Autodesk Fusion 360 part; units mm, degrees
sketch "Sketch1" plane through (0, 0, 0) normal (0, 0, 1) x (1, 0, 0)
  line L0 (-35, 30) -> (60, 30)
  line L1 (60, 30) -> (60, -52)
  line L2 (60, -52) -> (-35, -52)
  line L3 (-35, -52) -> (-35, 30)
  line L4 (-38, 33) -> (63, 33)
  line L5 (63, 33) -> (63, -55)
  line L6 (63, -55) -> (-38, -55)
  line L7 (-38, -55) -> (-38, 33)
  dimension "d1" = 82
  dimension "d2" = 95
  dimension "d3" = 3
  dimension "d4" = 3
  dimension "d5" = 3
  dimension "d6" = 3
extrude "Extrude1" add sketch "Sketch1" along normal blind 40
extrude "Extrude2" add sketch "Sketch1" along normal blind 4 contours L0 L1 L2 L3
sketch "Sketch2" plane through (63, 0, 0) normal (1, 0, 0) x (0, 1, 0)
  line L0 (-55, 0) -> (33, 0)
  line L1 (33, 0) -> (33, 40)
  line L2 (33, 40) -> (-55, 40)
  line L3 (-55, 40) -> (-55, 0)
  line L4 (-22, 29) -> (-40, 29)
  line L5 (-40, 29) -> (-40, 11)
  line L6 (-40, 11) -> (-22, 11)
  line L7 (-22, 11) -> (-22, 29)
  line L8 (-22, 29) -> (-40, 11) construction
  line L9 (-40, 29) -> (-22, 11) construction
  point P0 (-31, 20)
  dimension "d11" = 18
  dimension "d12" = 18
  dimension "d13" = 15
  dimension "d14" = 11
extrude "Extrude3" cut sketch "Sketch2" against normal blind 3 contours L4 L5 L6 L7
fillet "Fillet1" radius 2 1 edges at (63, -55, 20)
fillet "Fillet2" radius 2 1 edges at (63, 33, 20)
fillet "Fillet3" radius 2 1 edges at (-38, 33, 20)
fillet "Fillet4" radius 2 1 edges at (-38, -55, 20)
fillet "Fillet5" radius 2 1 edges at (-35, 30, 22)
fillet "Fillet6" radius 2 1 edges at (-35, -52, 22)
fillet "Fillet7" radius 2 1 edges at (60, -52, 22)
fillet "Fillet8" radius 2 1 edges at (60, 30, 22)
Geometry check sheet. Reference: the model listing, model coordinates, mm. A direction names the side the tool comes from. Coordinates: 2 decimals unless noted, no trailing zeros. Loops run counter-clockwise (first coordinate to the right, second up) from the corner with the lowest first, then second, coordinate; pieces in that order, holes last. Notation, with made-up numbers: (-31.75, -16.5) - (-2.75, -16.5) arc R37 cw to (-2.75, 22.5) - close; hole circle Ø9 at (-22, -38). An arc over 180 degrees is marked (long way). One line per item, written item: value. Start each with the question number.
(1) Tool access check on faces 1 (the flat face through (12, -10, 4)), 2 (the flat face through (62, -40, 20)), 3 (the flat face through (13, -55, 20)). Record the directions out of +Z, -Z, +X, -X, +Y, -Y that give a thin tool (end or side, any length) a straight path to the whole face; none if there is none.
(2) Cross-section at B-B on y = -36. Enter the section's corners in (x, z).
(3) Material ranges on line 1 (Y direction, x = -9, z = 20); line 2 (X direction, y = 4, z = 8); line 3 (Z direction, x = -33, y = -43.5), recorded low to high. Write a range as [from, to].
(4) Cross-section at C-C on x = -22. Enter the section's corners in (y, z).
(5) Depth check by flat-ended pin: P1, Ø10, axis at x = 44, y = -27.5, coming from the +Z side; P2, Ø0.9, axis at x = 62, z = 16, coming from the -Y side. Enter the tip coordinate at first touch or a pass-through.
(6) Mould release check, pull along X, two halves, no side actions. Record for faces 4 (the flat face through (62, -22, 20)), 5 (the flat face through (13, -52, 22)), 6 (the flat face through (-38, -12, 20)), 7 (the flat face through (63, -10, 20)): released by +X, released by -X, zero draft, split by the parting line, or undercut.
(7) Cross-section at D-D on y = 12.5. Enter the section's corners in (x, z), plus the area to 3 significant figures.
(8) Cross-section at A-A on z = 30.5. Enter the section's corners in (x, y).
Results below:
1. face 1: +Z
1. face 2: +X
1. face 3: +Z, -Z, +X, -X, -Y
2. outline: (-38, 0) - (63, 0) - (63, 11) - (60, 11) - (60, 4) - (-35, 4) - (-35, 40) - (-38, 40) - close; (60, 29) - (63, 29) - (63, 40) - (60, 40) - close
3. line 1: y = [-55, -52], [30, 33]
3. line 2: x = [-38, -35], [60, 63]
3. line 3: z = [0, 4]
4. outline: (-55, 0) - (33, 0) - (33, 40) - (30, 40) - (30, 4) - (-52, 4) - (-52, 40) - (-55, 40) - close
5. P1: stops at z = 4
5. P2: stops at y = -54.92
6. face 4: zero draft
6. face 5: undercut
6. face 6: released by -X
6. face 7: released by +X
7. outline: (-38, 0) - (63, 0) - (63, 40) - (60, 40) - (60, 4) - (-35, 4) - (-35, 40) - (-38, 40) - close
7. area: 620 mm2
8. outline: (-38, -53) arc R2 ccw to (-36, -55) - (61, -55) arc R2 ccw to (63, -53) - (63, 31) arc R2 ccw to (61, 33) - (-36, 33) arc R2 ccw to (-38, 31) - close; hole (-35, -50) arc R2 ccw to (-33, -52) - (58, -52) arc R2 ccw to (60, -50) - (60, 28) arc R2 ccw to (58, 30) - (-33, 30) arc R2 ccw to (-35, 28) - close
